```python
from build123d import *

# Parameters (mm, degrees)
F0_R     = 5.8
F0_R_2   = 4.8
F1_DEPTH = 1
F2_DEPTH = 3.8
F3_R     = 1.2
F4_DEPTH = 1


with BuildPart() as f1:
    # F0 (on Front) → F1 (new body)
    with BuildSketch(Plane.XZ):
        Circle(F0_R)
        Circle(F0_R_2, mode=Mode.SUBTRACT)
        Circle(F0_R_2)
    extrude(amount=F1_DEPTH)

    # F0 (on Front) → F2 (join)
    with BuildSketch(Plane.XZ):
        Circle(F0_R_2)
    extrude(amount=F2_DEPTH)

    # F3 (on face) → F4 (join)
    with BuildSketch(Plane.XZ):
        Circle(F3_R)
    extrude(amount=-F4_DEPTH)


solid = f1.part
```
Verification items for the finished model (mm, model axes). A direction names the side the tool comes from. Coordinates: 2 decimals unless noted, no trailing zeros. Loops run counter-clockwise (first coordinate to the right, second up) from the corner with the lowest first, then second, coordinate; pieces in that order, holes last. Notation, with made-up numbers: (53.25, -38) -> (110.25, -38) arc R18 cw to (110.25, -33) -> close; hole circle Ø2 at (-28.75, -25.5). An arc over 180 degrees is marked (long way). Put each result on its own line as item: value.
1. Thickness scan on line 1 (Y direction, x = -2.5, z = -1); line 2 (Z direction, x = 0, y = -2.9); line 3 (Y direction, x = -5, z = -1.5). Record the ranges inside material, lowest first.
Result set:
line 1: y = -3.8 to 0
line 2: z = -4.8 to 4.8
line 3: y = -1 to 0
2. Section check C-C, the plane y = -2.85. Record the boundary of the cut face in (x, z).
Result set:
outline: circle Ø9.6 at (0, 0)
3. Tool access check on faces 1 (the face through (1, -1, 5)), 2 (the face through (0, 1, 0)), 3 (the face through (0.65, 0.49, 1.01)). Record the directions out of +Z, -Z, +X, -X, +Y, -Y that give a thin tool (end or side, any length) a straight path to the whole face; none if there is none.
Result set:
face 1: -Y
face 2: +Z, -Z, +X, -X, +Y
face 3: +Y
4. Gauge pin test, flat ends, axial feed: P1, Ø3, axis at x = 1.5, z = 1, coming from the +Y side; P2, Ø1, axis at x = -4, y = -1, coming from the +Z side. Record the tip position at first contact, or that the pin passes through.
Result set:
P1: stops at y = 1
P2: stops at z = 4.62
5. Section check B-B, the plane x = 0. Record the boundary of the cut face in (y, z), then the cut area to 3 significant figures.
Result set:
outline: (-3.8, -4.8) -> (-1, -4.8) -> (-1, -5.8) -> (0, -5.8) -> (0, -1.2) -> (1, -1.2) -> (1, 1.2) -> (0, 1.2) -> (0, 5.8) -> (-1, 5.8) -> (-1, 4.8) -> (-3.8, 4.8) -> close
area: 40.9 mm^2
6. Section check D-D, the plane x = -3.75. Record the boundary of the cut face in (y, z), then the cut area to 3 significant figures.
Result set:
outline: (-3.8, -3) -> (-1, -3) -> (-1, -4.42) -> (0, -4.42) -> (0, 4.42) -> (-1, 4.42) -> (-1, 3) -> (-3.8, 3) -> close
area: 25.6 mm^2
7. Section check A-A, the plane z = 0. Record the boundary of the cut face in (x, y), then the cut area to 3 significant figures.
Result set:
outline: (-5.8, -1) -> (-4.8, -1) -> (-4.8, -3.8) -> (4.8, -3.8) -> (4.8, -1) -> (5.8, -1) -> (5.8, 0) -> (1.2, 0) -> (1.2, 1) -> (-1.2, 1) -> (-1.2, 0) -> (-5.8, 0) -> close
area: 40.9 mm^2
